from build123d import *

# Parameters (mm, degrees)
SKETCH1_W           = 85
SKETCH1_H           = 67
BOSS_EXTRUDE1_DEPTH = 4
SKETCH2_R           = 1.5
CUT_EXTRUDE1_DEPTH  = 4
SKETCH3_R           = 1.5
SKETCH3_R_2         = 1.67
CUT_EXTRUDE2_DEPTH  = 10


with BuildPart() as part:
    # Sketch1 → Boss-Extrude1 (new body)
    with BuildSketch(Plane(origin=(0, 0, 0), x_dir=(1, 0, 0), z_dir=(0, 1, 0))):
        Rectangle(SKETCH1_W, SKETCH1_H)
    extrude(amount=BOSS_EXTRUDE1_DEPTH)

    # Sketch2 → Cut-Extrude1 (cut)
    with BuildSketch(Plane(origin=(0, 4, 0), x_dir=(1, 0, 0), z_dir=(0, 1, 0))):
        with Locations(Location((-40.125, 20.85, 0), (0, 0, 270))):
            Circle(SKETCH2_R)
        with Locations(Location((-40.125, -20.85, 0), (0, 0, 270))):
            Circle(SKETCH2_R)
        with Locations(Location((40.125, 20.85, 0), (0, 0, 270))):
            Circle(SKETCH2_R)
        with Locations(Location((40.125, -20.85, 0), (0, 0, 270))):
            Circle(SKETCH2_R)
    extrude(amount=-CUT_EXTRUDE1_DEPTH, mode=Mode.SUBTRACT)

    # Sketch3 → Cut-Extrude2 (cut)
    with BuildSketch(Plane(origin=(0, 4, 0), x_dir=(1, 0, 0), z_dir=(0, 1, 0))):
        with Locations(Location((26.173152267, 20.95, 0), (0, 0, 270))):
            Circle(SKETCH3_R)
        with Locations(Location((26.173152267, -20.95, 0), (0, 0, 270))):
            Circle(SKETCH3_R)
        with Locations(Location((-38.73, 26, 0), (0, 0, 270))):
            Circle(SKETCH3_R_2)
        with Locations(Location((-38.73, -26, 0), (0, 0, 270))):
            Circle(SKETCH3_R)
    extrude(amount=-CUT_EXTRUDE2_DEPTH, mode=Mode.SUBTRACT)


solid = part.part
CAD build for the part. Positions are in the model's coordinates, mm. Coordinates: 2 decimals unless noted, no trailing zeros. Write each loop counter-clockwise with the first axis right and the second up, starting at its lowest first coordinate (ties: lowest second). Pieces come first, ordered by that corner, then holes. Notation, with made-up numbers: M -17.75,55.25 L 31.25,55.25 A27 cw 31.25,91.25 Z; hole C 69,8 d7. An arc over 180 degrees is marked long. Return JSON: item names as keys, results as strings.
Item 1: Two-plate mould, pull along Z, no slides. Class faces 1 (the cylindrical face through (38.794, 2.028, -20.158)), 2 (the flat face through (-1, 0, 0)), 3 (the cylindrical face through (27.66, 2.03, 20.75)), 4 (the flat face through (-1, 2, -33.5)): +Z half, -Z half, draft (parallel to the pull), parting line (faces both ways), or undercut.
Findings below:
{"face 1": "undercut", "face 2": "draft", "face 3": "undercut", "face 4": "-Z half"}
Item 2: Slice it at A-A, the plane z = 26. Write the cut outline in (x, y).
Findings below:
{"outline": "M -42.5,0 L -40.23,0 L -40.23,4 L -42.5,4 Z; M -37.23,0 L 42.5,0 L 42.5,4 L -37.23,4 Z"}
Item 3: Probe line 1 (X direction, y = 2.5, z = -20.95); line 2 (X direction, y = 1.95, z = 26); line 3 (Z direction, x = 39, y = 2.4). List the from-to ranges inside material, lowest first. Write a range as from..to.
Findings below:
{"line 1": "x = -42.5..-41.62, -38.63..24.67, 27.67..38.63, 41.62..42.5", "line 2": "x = -42.5..-40.23, -37.23..42.5", "line 3": "z = -33.5..-21.84, -19.86..19.86, 21.84..33.5"}
